```python
from build123d import *

# Parameters (mm, degrees)
EXTRUDE_1_DEPTH     = 6
SKETCH_3_R          = 2.5
CUT_EXTRUDE_1_DEPTH = 50.437261579


with BuildPart() as part:
    # Эскиз1 → Бобышка-Вытянуть1 (new body)
    with BuildSketch(Plane.XY):
        with BuildLine():
            ThreePointArc((18.964860111, 23.850911821), (0, 37.5), (-18.964860111, 23.850911821))
            Line((-18.964860111, 23.850911821), (-31.004148648, -12.100370354))
            ThreePointArc((-31.004148648, -12.100370354), (-29.296713539, -23.371522252), (-19.151111078, -28.569690242))
            Line((-19.151111078, -28.569690242), (19.151111078, -28.569690242))
            ThreePointArc((19.151111078, -28.569690242), (29.296713539, -23.371522252), (31.004148648, -12.100370354))
            Line((31.004148648, -12.100370354), (18.964860111, 23.850911821))
        make_face()
    extrude(amount=EXTRUDE_1_DEPTH)

    # Эскиз3 → Вырез-Вытянуть1 (cut, through all)
    with BuildSketch(Plane.XY.offset(6)):
        Circle(SKETCH_3_R)
    extrude(amount=-CUT_EXTRUDE_1_DEPTH, mode=Mode.SUBTRACT)


solid = part.part
```
Build history of the part. All positions in model axes, mm. Round coordinates to 2 decimals unless told otherwise and drop trailing zeros. Order: outer loops, then holes, each group sorted by start corner. A loop starts at its lowest first (then second) coordinate and runs counter-clockwise, first axis right, second up. Notation, with made-up numbers: (20.25, 44.5) -> (58.25, 44.5) arc R14 cw to (58.25, 56.5) -> close; hole circle Ø5 at (-18, 63). An arc over 180 degrees is marked (long way). Answer in a Markdown table with one row per item.
1) Band-saw the part on A-A on x = 0. Give the cut face in (y, z).
Values:
| item | result |
|---|---|
| outline | (-28.57, 0) -> (-2.5, 0) -> (-2.5, 6) -> (-28.57, 6) -> close; (2.5, 0) -> (37.5, 0) -> (37.5, 6) -> (2.5, 6) -> close |
2) Mould opens along Y. For faces 1 (the flat face through (-24.9, 6.13, 2.96)), 2 (the cylindrical face through (-0.54, -2.44, 3.04)), 3 (the flat face through (0, 5, 6)) say: released by +Y, released by -Y, zero draft, split by the parting line, or undercut.
Values:
| item | result |
|---|---|
| face 1 | released by +Y |
| face 2 | undercut |
| face 3 | zero draft |
3) Band-saw the part on C-C on y = 0. Give the cut face in (x, z), and give its area (3 significant figures).
Values:
| item | result |
|---|---|
| outline | (-26.95, 0) -> (-2.5, 0) -> (-2.5, 6) -> (-26.95, 6) -> close; (2.5, 0) -> (26.95, 0) -> (26.95, 6) -> (2.5, 6) -> close |
| area | 293 mm2 |
4) Band-saw the part on B-B on z = 2.4. Give the cut face in (x, y), and give its area (3 significant figures).
Values:
| item | result |
|---|---|
| outline | (-31, -12.1) arc R12.5 ccw to (-19.15, -28.57) -> (19.15, -28.57) arc R12.5 ccw to (31, -12.1) -> (18.96, 23.85) arc R20 ccw to (-18.96, 23.85) -> close; hole circle Ø5 at (0, 0) |
| area | 3,130 mm2 |
5) Band-saw the part on D-D on y = 29.5. Give the cut face in (x, z).
Values:
| item | result |
|---|---|
| outline | (-16, 0) -> (16, 0) -> (16, 6) -> (-16, 6) -> close |
6) Pin check, flat tips, straight feed: P1, Ø1, axis at y = 25, z = 3.5, coming from the -X side (3 decimals); P2, Ø1, axis at x = 8.5, z = 1.5, coming from the +Y side. Stop position of each tip, or through.
Values:
| item | result |
|---|---|
| P1 | x = -18.735 |
| P2 | y = 35.83 |
7) Wall check: L1, parallel to Y at x = 0, z = 2.45; L2, parallel to X at y = 1.5, z = 3.4; L3, parallel to X at y = 27, z = 5.45. Give the ranges that are in metal, low to high.
Values:
| item | result |
|---|---|
| L1 | -28.57 to -2.5, 2.5 to 37.5 |
| L2 | -26.45 to -2, 2 to 26.45 |
| L3 | -17.6 to 17.6 |
